Could you check a few things on this model? Use its own coordinates, in mm. A direction names the side the tool comes from. Coordinates: 2 decimals unless noted, no trailing zeros. Loops run counter-clockwise (first coordinate to the right, second up) from the corner with the lowest first, then second, coordinate; pieces in that order, holes last. Notation, with made-up numbers: M -38,-9 L -15,-9 A17 cw -15,1 Z; hole C 86,53.25 d8. An arc over 180 degrees is marked long. Write each question's results on one line, items separated by ' | '.
```python
from build123d import *

# Parameters (mm, degrees)
SKETCH1_W              = 95.8
SKETCH1_H              = 44.8
MAINWALL_DEPTH         = 10
SKETCH2_R              = 3
SPRINGAXLE_DEPTH       = 23
SKETCH3_R              = 5.75
SPOOLSUPPORTAXLE_DEPTH = 5
SKETCH4_W              = 0.2
SKETCH4_H              = 20
SLICE_2_DEPTH          = 18
FILLET1_R              = 0.5


with BuildPart() as part:
    # Sketch1 → MainWall (new body)
    with BuildSketch(Plane.XY):
        Rectangle(SKETCH1_W, SKETCH1_H)
    extrude(amount=MAINWALL_DEPTH)

    # Sketch2 → SpringAxle (add)
    with BuildSketch(Plane.XY.offset(10)):
        with Locations((18.75, 0)):
            Circle(SKETCH2_R)
    extrude(amount=SPRINGAXLE_DEPTH)

    # Sketch3 → SpoolSupportAxle (add)
    with BuildSketch(Plane.XY.offset(10)):
        with Locations((18.75, 0)):
            Circle(SKETCH3_R)
    extrude(amount=SPOOLSUPPORTAXLE_DEPTH)

    # Sketch4 → Slice 2 (cut)
    with BuildSketch(Plane.XY.offset(33)):
        with Locations((18.75, 0)):
            Rectangle(SKETCH4_W, SKETCH4_H)
    extrude(amount=-SLICE_2_DEPTH, mode=Mode.SUBTRACT)

    # Fillet1
    fillet1_edges = [part.edges().sort_by_distance(p)[0] for p in [
        (13, 0, 15),
        (15.75, 0, 33),
        (21.75, 0, 33),
        (18.85, 0, 33),
        (18.65, 0, 33),
    ]]
    fillet(fillet1_edges, radius=FILLET1_R)


solid = part.part
```
(1) If we mould it in two halves opening along X, with no side actions, what happens to faces 1 (the flat face through (-1, -22.4, 5)), 2 (the flat face through (47.9, 0, 5)), 3 (the flat face through (18.65, 0, 24))? For each: released by +X, released by -X, zero draft, split by the parting line, or undercut.
Reported:
face 1: zero draft | face 2: released by +X | face 3: undercut
(2) Please list where these lines run through material, in increasing order: probe 1 along Z at (x, y) = (-8, -19); probe 2 along X at (y, z) = (0.5, 18); probe 3 along X at (y, z) = (3.5, 13.5). Write a range as from..to.
Reported:
probe 1: z = 0..10 | probe 2: x = 15.79..18.65, 18.85..21.71 | probe 3: x = 14.19..23.31
(3) Imagine slicing it at D-D, the plane z = 13. List the corners of the cut face in (x, y) for me.
Reported:
outline: C 18.75,0 d11.5
(4) Will these pins go through, and if not, where does the flat tip stop? P1, Ø12, axis at x = -28.5, z = 21.5, coming from the -Y side; P2, Ø22.5, axis at x = -7, y = -6, coming from the +Z side; P3, Ø10, axis at y = 7, z = 24, coming from the +X side; P4, Ø6.5, axis at y = -0.5, z = 22.5, coming from the +X side.
Reported:
P1: passes through | P2: stops at z = 10 | P3: stops at x = 20.99 | P4: stops at x = 21.75
(5) Which directions (+Z, -Z, +X, -X, +Y, -Y) give clear straight access to the entire face, cutting with the end or side of a thin tool? Please do faces 4 (the flat face through (17, 0, 33)), 5 (the flat face through (18.85, 0, 24)), 6 (the cylindrical face through (15.75, 0.06, 23.63)), 7 (the cylindrical face through (21.75, -0.06, 23.63)), 8 (the flat face through (21, -2.3, 15)).
Reported:
face 4: +Z, +X, -X, +Y, -Y | face 5: +Z, +Y, -Y | face 6: +Z, -X | face 7: +Z, +X | face 8: +Z
(6) Imagine slicing it at A-A, the plane y = 0. List the corners of the cut face in (x, z) for me.
Reported:
outline: M -47.9,0 L 47.9,0 L 47.9,10 L 24.5,10 L 24.5,14.5 A0.5 ccw 24,15 L 21.75,15 L 21.75,32.5 A0.5 ccw 21.25,33 L 19.35,33 A0.5 ccw 18.85,32.5 L 18.85,15 L 18.65,15 L 18.65,32.5 A0.5 ccw 18.15,33 L 16.25,33 A0.5 ccw 15.75,32.5 L 15.75,15 L 13.5,15 A0.5 ccw 13,14.5 L 13,10 L -47.9,10 Z
(7) Imagine slicing it at C-C, the plane x = -17. List the corners of the cut face in (y, z) for me, and give its area (3 significant figures).
Reported:
outline: M -22.4,0 L 22.4,0 L 22.4,10 L -22.4,10 Z | area: 448 mm2
